Input: dimensioned drawing with shaded views. Units: mm. Origin: part minimum x, y, z. Give positions to 0.01 mm unless a question says otherwise; leave off trailing zeros. Loops run counter-clockwise (first coordinate to the right, second up) from the corner with the lowest first, then second, coordinate; pieces in that order, holes last.
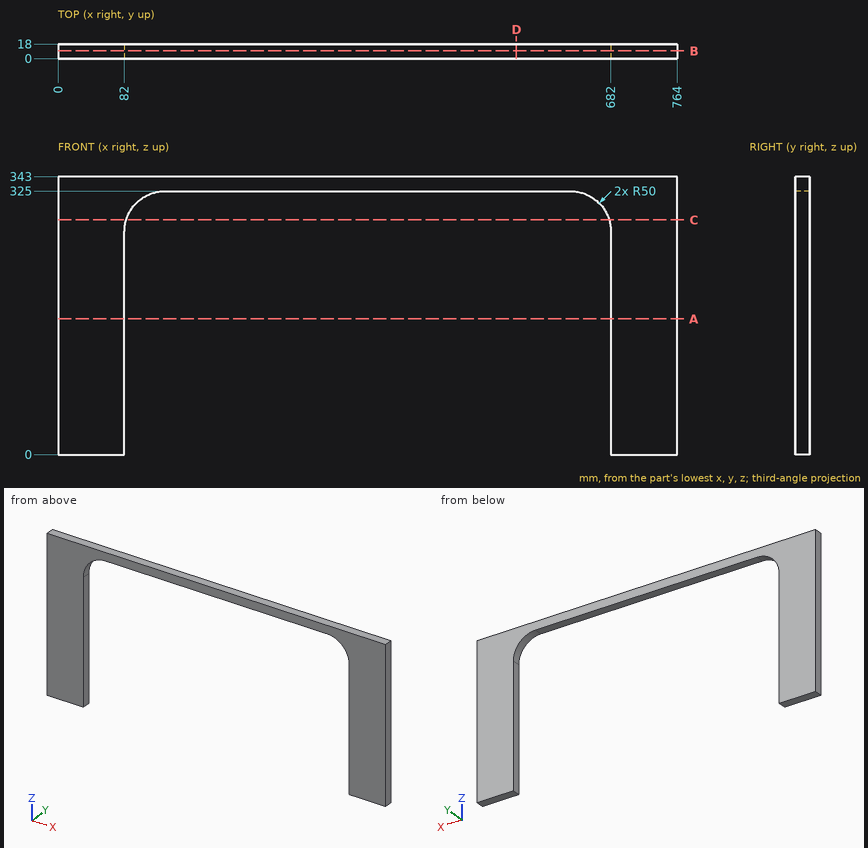
(1) Ray query, line 1 along X through (y, z) = (5, 278); line 2 along X through (y, z) = (13.75, 135.5); line 3 along Z through (x, y) = (155, 7.75). Return the intervals inside material, ascending.
A:
line 1: x = 0 to 82.09, 681.91 to 764
line 2: x = 0 to 82, 682 to 764
line 3: z = 325 to 343
(2) Section A-A, the plane z = 167.5. Return the cut outline in (x, y), then the cut area to 3 significant figures.
A:
outline: (0, 0) - (82, 0) - (82, 18) - (0, 18) - close; (682, 0) - (764, 0) - (764, 18) - (682, 18) - close
area: 2,950 mm2
(3) First-contact query: pin 1 (5 mm diameter, centred on x = 518.5, y = 3.5, fed in from -Z). Flat tip, straight axial feed; report the tip coordinate or a pass-through.
A:
pin 1: stops at z = 325
(4) Section C-C, the plane z = 289.5. Return the cut outline in (x, y), then the cut area to 3 significant figures.
A:
outline: (0, 0) - (84.15, 0) - (84.15, 18) - (0, 18) - close; (679.85, 0) - (764, 0) - (764, 18) - (679.85, 18) - close
area: 3,030 mm2
(5) Section B-B, the plane y = 9.5. Return the cut outline in (x, z), then the cut area to 3 significant figures.
A:
outline: (0, 0) - (82, 0) - (82, 275) arc R50 cw to (132, 325) - (632, 325) arc R50 cw to (682, 275) - (682, 0) - (764, 0) - (764, 343) - (0, 343) - close
area: 68,100 mm2
(6) Section D-D, the plane x = 565.5. Return the cut outline in (y, z), then the cut area to 3 significant figures.
A:
outline: (0, 325) - (18, 325) - (18, 343) - (0, 343) - close
area: 324 mm2
